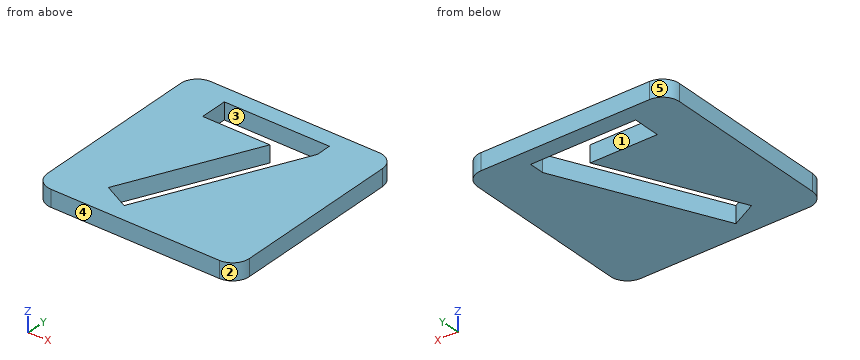
```python
from build123d import *

# Parameters (mm, degrees)
BOSS_EXTRUDE1_DEPTH = 10
CUT_EXTRUDE6_DEPTH  = 10


with BuildPart() as part:
    # Sketch1 → Boss-Extrude1 (new body)
    with BuildSketch(Plane.XY):
        with BuildLine():
            Line((-50, 60), (50, 60))
            ThreePointArc((50, 60), (57.071067812, 57.071067812), (60, 50))
            Line((60, 50), (60, -50))
            ThreePointArc((60, -50), (57.071067812, -57.071067812), (50, -60))
            Line((50, -60), (-50, -60))
            ThreePointArc((-50, -60), (-57.071067812, -57.071067812), (-60, -50))
            Line((-60, -50), (-60, 50))
            ThreePointArc((-60, 50), (-57.071067812, 57.071067812), (-50, 60))
        make_face()
    extrude(amount=BOSS_EXTRUDE1_DEPTH)

    # Sketch2 → Cut-Extrude6 (cut)
    with BuildSketch(Plane.XY.offset(10)):
        Polygon((-34, 50), (28.5, 50), (28.5, 40.91796875), (-14.5078125, -50), (-30.015625, -42.1875), (5.921875, 33.75), (-34, 33.75), align=None)
    extrude(amount=-CUT_EXTRUDE6_DEPTH, mode=Mode.SUBTRACT)


solid = part.part
```
For this review, take the finished solid that the model builds, in its own axes (mm). Face numbers are marked on the shaded views. A direction names the side the tool comes from. Round coordinates to 2 decimals unless told otherwise and drop trailing zeros. Write each loop counter-clockwise with the first axis right and the second up, starting at its lowest first coordinate (ties: lowest second). Pieces come first, ordered by that corner, then holes.
1) Machinability: for the marked faces 1 and 2, which of the approach directions +Z, -Z, +X, -X, +Y, -Y give a long, thin tool a straight path to every point of the face, cutting with its end or side? Answer none if there is none.
Answer below:
face 1: +Z, -Z
face 2: +Z, -Z, +X, -Y
2) Take a section at B-B on y = 27. Give the boundary of the cut face in (x, z).
Answer below:
outline: (-60, 0) - (2.73, 0) - (2.73, 10) - (-60, 10) - close; (21.92, 0) - (60, 0) - (60, 10) - (21.92, 10) - close
3) Insertion check: pin 1 Ø3 at (x, y) = (22, 28) entering from -Z. The pin has a flat end and moves straight along its axis. Give the tip position at first contact, or say it passes through.
Answer below:
pin 1: stops at z = 0
4) Take a section at A-A on z = 6. Give the boundary of the cut face in (x, y), then the cut area to 3 significant figures.
Answer below:
outline: (-60, -50) arc R10 ccw to (-50, -60) - (50, -60) arc R10 ccw to (60, -50) - (60, 50) arc R10 ccw to (50, 60) - (-50, 60) arc R10 ccw to (-60, 50) - close; hole (-34, 33.75) - (5.92, 33.75) - (-30.02, -42.19) - (-14.51, -50) - (28.5, 40.92) - (28.5, 50) - (-34, 50) - close
area: 11,800 mm2
5) Take a section at D-D on x = -16. Give the boundary of the cut face in (y, z).
Answer below:
outline: (-60, 0) - (-49.25, 0) - (-49.25, 10) - (-60, 10) - close; (-12.57, 0) - (33.75, 0) - (33.75, 10) - (-12.57, 10) - close; (50, 0) - (60, 0) - (60, 10) - (50, 10) - close
6) For line 1 along Y through (x, z) = (-7.5, 1.75); line 2 along Y through (x, z) = (-33.5, 7); line 3 along Y through (x, z) = (-19.5, 4.5), list the stretches that pass through material, from the lowest coordinate up.
Answer below:
line 1: y = -60 to -35.19, 5.39 to 33.75, 50 to 60
line 2: y = -60 to 33.75, 50 to 60
line 3: y = -60 to -47.49, -19.97 to 33.75, 50 to 60
7) Mouldability with a two-part tool opening along X and no side actions: class the marked faces 3, 4 and 5 as +X half, -X half, draft (parallel to the pull), parting line (faces both ways), or undercut.
Answer below:
face 3: undercut
face 4: draft
face 5: -X half
8) Take a section at C-C on x = -4. Give the boundary of the cut face in (y, z).
Answer below:
outline: (-60, 0) - (-27.79, 0) - (-27.79, 10) - (-60, 10) - close; (12.78, 0) - (33.75, 0) - (33.75, 10) - (12.78, 10) - close; (50, 0) - (60, 0) - (60, 10) - (50, 10) - close
